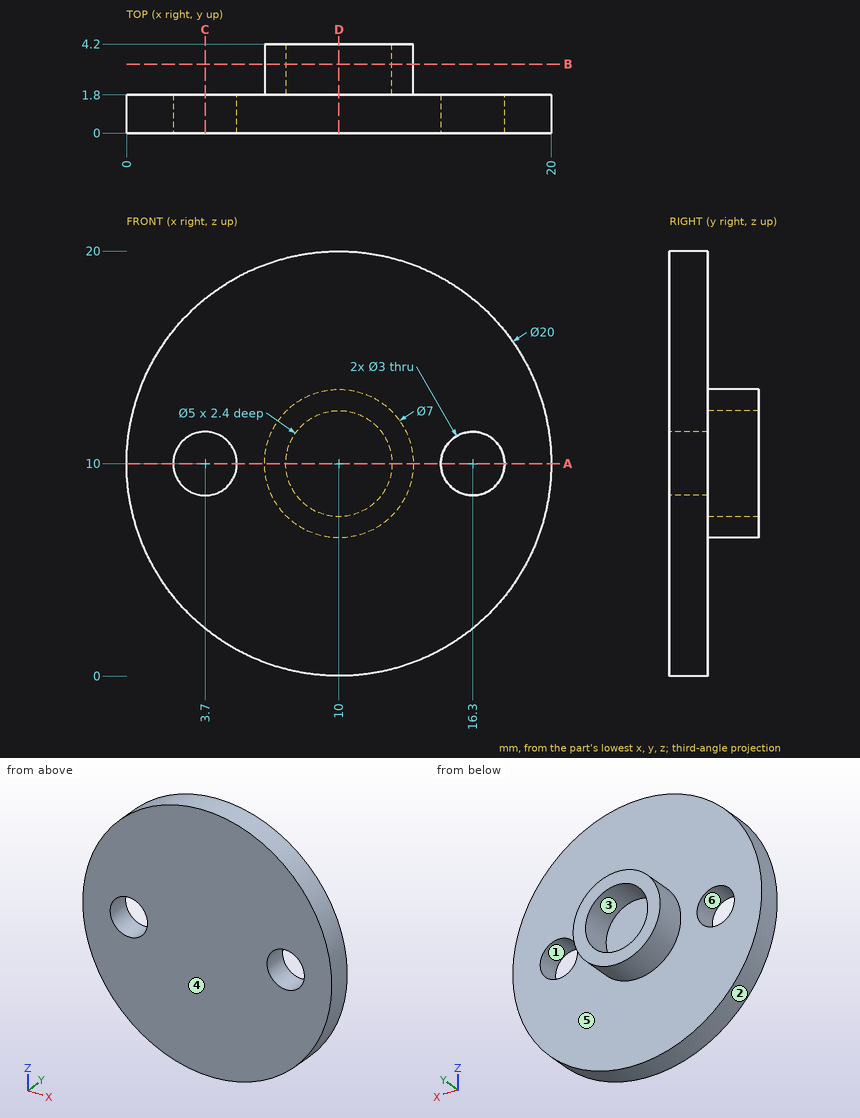
Could you check a few things on this drawing? It's one solid part, dimensions in mm from its lowest x, y, z. A direction names the side the tool comes from. Coordinates: 2 decimals unless noted, no trailing zeros. Order: outer loops, then holes, each group sorted by start corner. A loop starts at its lowest first (then second) coordinate and runs counter-clockwise, first axis right, second up. Notation, with made-up numbers: (21.25, 49.5) -> (55.25, 49.5) arc R15 cw to (55.25, 53.5) -> close; hole circle Ø10 at (16, -1). An arc over 180 degrees is marked (long way). Answer in a Markdown table with one row per item.
(1) Will these pins go through, and if not, where does the flat tip stop? pin 1 Ø1 at (x, y) = (12, 1) entering from -Z; pin 2 Ø1 at (y, z) = (2, 3) entering from +X; pin 3 Ø4 at (x, z) = (3.7, 10) entering from +Y.
Answer key:
| item | result |
|---|---|
| pin 1 | z = 0.11 |
| pin 2 | x = 17.56 |
| pin 3 | y = 1.8 |
(2) I want a section at D-D on x = 10. List the corners of the cut face in (y, z) for me, then the cut area to 3 significant figures.
Answer key:
| item | result |
|---|---|
| outline | (0, 0) -> (1.8, 0) -> (1.8, 6.5) -> (4.2, 6.5) -> (4.2, 7.5) -> (1.8, 7.5) -> (1.8, 12.5) -> (4.2, 12.5) -> (4.2, 13.5) -> (1.8, 13.5) -> (1.8, 20) -> (0, 20) -> close |
| area | 40.8 mm^2 |
(3) Please list where these lines run through material, in increasing order: probe 1 along Z at (x, y) = (10, 2.5); probe 2 along X at (y, z) = (0.6, 10.25).
Answer key:
| item | result |
|---|---|
| probe 1 | 6.5 to 7.5, 12.5 to 13.5 |
| probe 2 | 0 to 2.22, 5.18 to 14.82, 17.78 to 20 |
(4) On a 3-axis mill with a long thin cutter (end or side, diameter ignored), from which of +Z, -Z, +X, -X, +Y, -Y can I reach the whole of each face in a straight line? I mean the marked faces 5 and 6. Say none if no direction works.
Answer key:
| item | result |
|---|---|
| face 5 | +Y |
| face 6 | +Y, -Y |
(5) I want a section at B-B on y = 3.25. List the corners of the cut face in (x, z) for me, then the cut area to 3 significant figures.
Answer key:
| item | result |
|---|---|
| outline | circle Ø7 at (10, 10); hole circle Ø5 at (10, 10) |
| area | 18.8 mm^2 |
(6) I want a section at A-A on z = 10. List the corners of the cut face in (x, y) for me.
Answer key:
| item | result |
|---|---|
| outline | (0, 0) -> (2.2, 0) -> (2.2, 1.8) -> (0, 1.8) -> close; (5.2, 0) -> (14.8, 0) -> (14.8, 1.8) -> (13.5, 1.8) -> (13.5, 4.2) -> (12.5, 4.2) -> (12.5, 1.8) -> (7.5, 1.8) -> (7.5, 4.2) -> (6.5, 4.2) -> (6.5, 1.8) -> (5.2, 1.8) -> close; (17.8, 0) -> (20, 0) -> (20, 1.8) -> (17.8, 1.8) -> close |
(7) I want a section at C-C on x = 3.7. List the corners of the cut face in (y, z) for me.
Answer key:
| item | result |
|---|---|
| outline | (0, 2.23) -> (1.8, 2.23) -> (1.8, 8.5) -> (0, 8.5) -> close; (0, 11.5) -> (1.8, 11.5) -> (1.8, 17.77) -> (0, 17.77) -> close |
(8) Thinking about a two-plate mould opening in Z: for the marked faces 1, 2, 3 and 4, which applies, +Z half, -Z half, draft (parallel to the pull), parting line (faces both ways), or undercut?
Answer key:
| item | result |
|---|---|
| face 1 | undercut |
| face 2 | parting line |
| face 3 | undercut |
| face 4 | draft |
